```python
from build123d import *

# Parameters (mm, degrees)
BOSS_EXTRUDE2_DEPTH      = 12.7
BOSS_EXTRUDE3_DEPTH      = 63.5
BOSS_EXTRUDE3_DEPTH_BACK = 51.59375
SKETCH3_R                = 12.7
CRVPATTERN3_START        = 25.4
CRVPATTERN3_OUTLINE_R    = 12.7
CRVPATTERN3_DEPTH        = 12.7
BOSS_EXTRUDE5_START      = -25.4
SKETCH7_R                = 22.225
BOSS_EXTRUDE5_DEPTH      = 4.7625
BOSS_EXTRUDE7_START      = -13.49375
SKETCH10_R               = 15.875
BOSS_EXTRUDE7_DEPTH      = 3.175
SKETCH9_R                = 7.9375
BOSS_EXTRUDE8_DEPTH      = 12.7


# Read off the part's stored shape, not the designer's step: CrvPattern3
with BuildPart() as part:
    # Sketch2 → Boss-Extrude2 (new body)
    with BuildSketch(Plane.XY):
        with BuildLine():
            ThreePointArc((-10.74656161, 14.203426928), (-11.786721082, 10.450325862), (-13.330377698, 6.874738694))
            ThreePointArc((-13.330377698, 6.874738694), (0, -14.9987), (13.330377698, 6.874738694))
            ThreePointArc((13.330377698, 6.874738694), (11.786721082, 10.450325862), (10.74656161, 14.203426928))
            ThreePointArc((10.74656161, 14.203426928), (0, 22.9743), (-10.74656161, 14.203426928))
        make_face()
    extrude(amount=BOSS_EXTRUDE2_DEPTH)

    # Sketch3 → Boss-Extrude3 (add, two sides: drawn at the far end of the back side and taken through both)
    with BuildSketch(Plane.XY.offset(12.7).offset(-BOSS_EXTRUDE3_DEPTH_BACK)):
        Circle(SKETCH3_R)
    extrude(amount=BOSS_EXTRUDE3_DEPTH + BOSS_EXTRUDE3_DEPTH_BACK)

    # CrvPattern3 outline → CrvPattern3 (add)
    with BuildSketch(Plane.XY.offset(CRVPATTERN3_START)):
        with BuildLine():
            ThreePointArc((6.874738694, 13.330377698), (-14.9987, 0), (6.874738694, -13.330377698))
            ThreePointArc((6.874738694, -13.330377698), (10.450325862, -11.786721082), (14.203426928, -10.74656161))
            ThreePointArc((14.203426928, -10.74656161), (22.9743, 0), (14.203426928, 10.74656161))
            ThreePointArc((14.203426928, 10.74656161), (10.450325862, 11.786721082), (6.874738694, 13.330377698))
        make_face()
        Circle(CRVPATTERN3_OUTLINE_R, mode=Mode.SUBTRACT)
    extrude(amount=CRVPATTERN3_DEPTH)

    # Sketch7 → Boss-Extrude5 (add)
    with BuildSketch(Plane.XY.offset(76.2).offset(BOSS_EXTRUDE5_START)):
        with Locations(Location((0, 0, 0), (0, 0, 180))):
            Circle(SKETCH7_R)
    extrude(amount=BOSS_EXTRUDE5_DEPTH)

    # Sketch10 → Boss-Extrude7 (add)
    with BuildSketch(Plane.XY.offset(76.2).offset(BOSS_EXTRUDE7_START)):
        Circle(SKETCH10_R)
    extrude(amount=-BOSS_EXTRUDE7_DEPTH)

    # Sketch9 → Boss-Extrude8 (add)
    with BuildSketch(Plane.XY.offset(76.2)):
        Circle(SKETCH9_R)
    extrude(amount=BOSS_EXTRUDE8_DEPTH)


solid = part.part
```
Work out the finished part from the listing and answer in its coordinate system (mm). A direction names the side the tool comes from. Coordinates: 2 decimals unless noted, no trailing zeros. Order: outer loops, then holes, each group sorted by start corner. A loop starts at its lowest first (then second) coordinate and runs counter-clockwise, first axis right, second up. Notation, with made-up numbers: M 35,-30 L 71,-30 A22 ccw 71,-3 Z; hole C 56.25,55.25 d5. An arc over 180 degrees is marked long. Use CSV: the item, a comma, the result in double quotes.
1) For faces 5 (the face through (11.805, 10.399, 6.261)), 6 (the face through (10.399, -11.805, 31.661)), 7 (the face through (-2.75, -12.4, -19.72)), 8 (the face through (-2.75, -12.4, 57.52)), determine the directions among +Z, -Z, +X, -X, +Y, -Y from which every point of the face is accessible in a straight line to the end or side of a thin tool.
Worked out:
face 5,"-Z, +X, +Y"
face 6,"-Z, +X, -Y"
face 7,"-Z"
face 8,"none"
2) Flat-ended cylindrical pins translate along their axes: pin 1 Ø2 at (y, z) = (-12.5, 21.5) entering from -X; pin 2 Ø6 at (x, y) = (-8, 8) entering from +Z; pin 3 Ø1 at (y, z) = (4.5, 23.5) entering from -X; pin 4 Ø9 at (x, y) = (10, 4) entering from +Z. Find the tip coordinate at first contact, or state that the pin passes through.
Worked out:
pin 1,"stops at x = -5.39"
pin 2,"stops at z = 76.2"
pin 3,"stops at x = -12.05"
pin 4,"stops at z = 88.9"
3) Section A-A on z = 71.5 is taken. Write down the section's boundary in (x, y).
Worked out:
outline,"C 0,0 d25.4"
4) Consider line 1 (Z direction, x = -4.5, y = -12.5); line 2 (Z direction, x = -15, y = 3); line 3 (Z direction, x = -17, y = 7). Determine where each line is inside the solid, lowest interval first. Write a range as [from, to].
Worked out:
line 1,"z = [0, 12.7], [25.4, 38.1], [50.8, 55.56], [59.53, 62.71]"
line 2,"z = [50.8, 55.56], [59.53, 62.71]"
line 3,"z = [50.8, 55.56]"
5) Determine the mould class of faces 1 (the face through (0, 0, 88.9)), 2 (the face through (-2.75, -12.4, 69.36)), 3 (the face through (3, 13, 0)), 4 (the face through (-7, 11, 59.531)) for opening direction Z: released by +Z, released by -Z, zero draft, split by the parting line, or undercut.
Worked out:
face 1,"released by +Z"
face 2,"zero draft"
face 3,"released by -Z"
face 4,"undercut"
